Answer from the drawing. Dimensions are ordinates in mm from the lowest x, y and z of the part. Coordinates: 2 decimals unless noted, no trailing zeros. Loops run counter-clockwise (first coordinate to the right, second up) from the corner with the lowest first, then second, coordinate; pieces in that order, holes last. Notation, with made-up numbers: (18.5, -24.5) -> (55.5, -24.5) arc R20 cw to (55.5, -13.5) -> close; hole circle Ø1 at (28, -18). An arc over 180 degrees is marked (long way). Use a Markdown table: item, result.
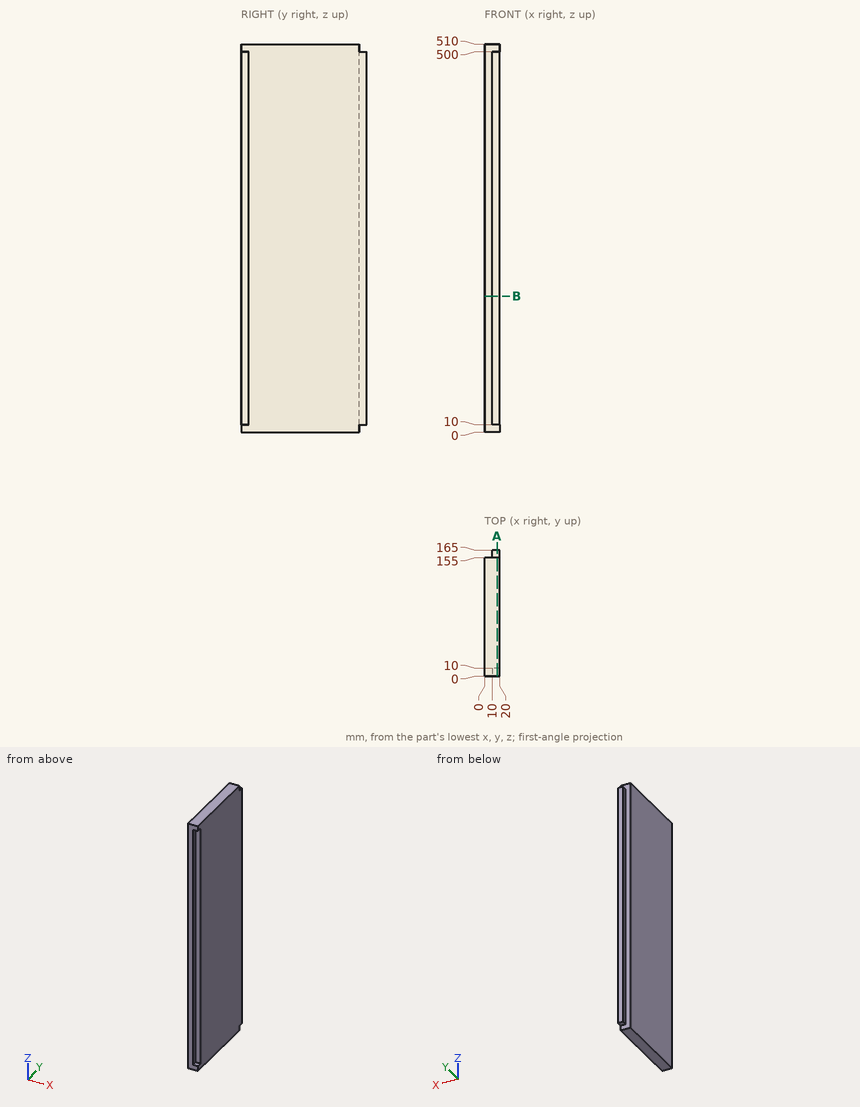
Q1. Section A-A on x = 16.25 is taken. Determine the outline of the cut face in (y, z).
Solved:
| item | result |
|---|---|
| outline | (0, 0) -> (155, 0) -> (155, 10) -> (165, 10) -> (165, 500) -> (155, 500) -> (155, 510) -> (0, 510) -> (0, 500) -> (10, 500) -> (10, 10) -> (0, 10) -> close |
Q2. Section B-B on z = 179 is taken. Determine the outline of the cut face in (x, y), and give its area (3 significant figures).
Solved:
| item | result |
|---|---|
| outline | (0, 0) -> (10, 0) -> (10, 10) -> (20, 10) -> (20, 165) -> (10, 165) -> (10, 155) -> (0, 155) -> close |
| area | 3,100 mm² |
Q3. Given pin 1 Ø8 at (x, y) = (15.5, 161) entering from -Z, flat-ended and moving along its own axis, determine where the tip first touches the part or whether it passes through.
Solved:
| item | result |
|---|---|
| pin 1 | z = 10 |
Q4. Consider line 1 (Y direction, x = 16, z = 270.5); line 2 (X direction, y = 9.5, z = 72); line 3 (Y direction, x = 2.5, z = 367). Determine where each line is inside the solid, lowest interval first. Write a range as [from, to].
Solved:
| item | result |
|---|---|
| line 1 | [10, 165] |
| line 2 | [0, 10] |
| line 3 | [0, 155] |
